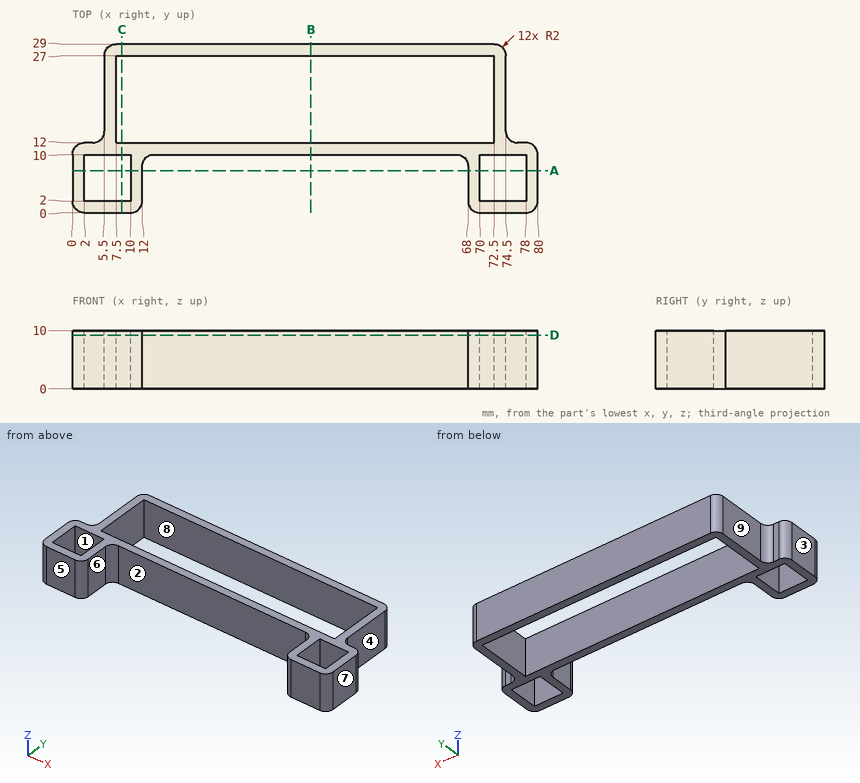
The figure shows three views and two pictorial views of one solid part (mm, origin at its lowest corner). Answer the questions. A direction names the side the tool comes from. Coordinates: 2 decimals unless noted, no trailing zeros. Loops run counter-clockwise (first coordinate to the right, second up) from the corner with the lowest first, then second, coordinate; pieces in that order, holes last.
1) Flat-ended cylindrical pins translate along their axes: pin 1 Ø0.8 at (x, z) = (3, 6) entering from +Y; pin 2 Ø3 at (x, z) = (38, 7) entering from -Y; pin 3 Ø3 at (y, z) = (17, 3) entering from +X. Find the tip coordinate at first contact, or state that the pin passes through.
2) A tool of negligible diameter and unlimited length cuts with its end or side. For the marked faces 1, 2, 3, 4 and 5, from which of +Z, -Z, +X, -X, +Y, -Y can it reach the whole face along a straight path? Write none if from no direction.
3) Determine the mould class of the marked faces 6, 7, 8 and 9 for opening direction X: pulls with the +X half, pulls with the -X half, needs draft (parallel to the pull), parting line crosses it, or undercut.
4) Find section A-A on y = 7.25. Write down the section's boundary in (x, z).
5) Find the intervals of material crossed by L1, parallel to X at y = 6.25, z = 7; L2, parallel to Y at x = 22, z = 7.25; L3, parallel to X at y = 9, z = 4.5, in increasing order.
6) Find section C-C on x = 8.5. Write down the section's boundary in (y, z), then the cut area to 3 significant figures.
7) Find section D-D on z = 9.25. Give the number of separate pieces and of enclosed holes in the cut face, then the cut area to 3 significant figures.
8) Find section B-B on x = 41. Write down the section's boundary in (y, z).
Values:
1. pin 1: stops at y = 12
1. pin 2: stops at y = 10
1. pin 3: stops at x = 74.5
2. face 1: +Z, -Z
2. face 2: +Z, -Z, -Y
2. face 3: +Z, -Z, -X, +Y, -Y
2. face 4: +Z, -Z, +X, +Y
2. face 5: +Z, -Z, +X, -X, -Y
3. face 6: undercut
3. face 7: pulls with the +X half
3. face 8: undercut
3. face 9: pulls with the -X half
4. outline: (0, 0) - (2, 0) - (2, 10) - (0, 10) - close; (10, 0) - (12, 0) - (12, 10) - (10, 10) - close; (68, 0) - (70, 0) - (70, 10) - (68, 10) - close; (78, 0) - (80, 0) - (80, 10) - (78, 10) - close
5. L1: x = 0 to 2, 10 to 12, 68 to 70, 78 to 80
5. L2: y = 10 to 12, 27 to 29
5. L3: x = 0 to 2, 10 to 12.27, 67.73 to 70, 78 to 80
6. outline: (0, 0) - (2, 0) - (2, 10) - (0, 10) - close; (10, 0) - (12, 0) - (12, 10) - (10, 10) - close; (27, 0) - (29, 0) - (29, 10) - (27, 10) - close
6. area: 60.0 mm2
7. separate pieces: 1
7. enclosed holes: 3
7. area: 467 mm2
8. outline: (10, 0) - (12, 0) - (12, 10) - (10, 10) - close; (27, 0) - (29, 0) - (29, 10) - (27, 10) - close
